Can you work these out from the model? Positions are in its coordinate system, mm. Face numbers are marked on the shaded views. A direction names the side the tool comes from. Round coordinates to 2 decimals unless told otherwise and drop trailing zeros. Write each loop counter-clockwise with the first axis right and the second up, starting at its lowest first coordinate (ties: lowest second). Pieces come first, ordered by that corner, then holes.
Q1. If we section it at C-C (z = 37): Please give me the cut outline in (x, y).
Q2. I'm going to push flat-ended pins straight in: pin 1 Ø19 at (x, y) = (12.5, -7) entering from +Z; pin 2 Ø4 at (x, y) = (-9, 20) entering from -Z; pin 3 Ø2 at (x, y) = (-31, -3.5) entering from +Z; pin 4 Ø8 at (x, y) = (13.5, 2.5) entering from +Z. Where does each tip first touch, or does it pass through?
Q3. Please list where these lines run through material, in increasing order: line 1 along Y through (x, z) = (-7, 8); line 2 along Y through (x, z) = (-3, 14); line 3 along X through (y, z) = (-17, 37.5).
Q4. For the marked faces 1 and 2, which set-ups out of +Z, -Z, +X, -X, +Y, -Y let a thin tool reach every point of the face, with its end or its side?
Q5. If we section it at D-D (x = -20.5): Please give me the cut outline in (y, z).
Q6. If we section it at A-A (x = 0): Please give me the cut outline in (y, z).
Q7. If we section it at B-B (y = 0): Please give me the cut outline in (x, z), plus the area to 3 significant figures.
from build123d import *

# Parameters (mm, degrees)
BOSS_EXTRUDE1_DEPTH = 40
FILLET1_R           = 4
SKETCH2_R           = 30
BOSS_EXTRUDE2_DEPTH = 4
SKETCH3_R           = 13.5
BOSS_EXTRUDE3_DEPTH = 44.5


with BuildPart() as part:
    # Sketch1 → Boss-Extrude1 (new, symmetric)
    with BuildSketch(Plane(origin=(0, 0, 0), x_dir=(0, 0, -1), z_dir=(1, 0, 0))):
        Polygon((0, 32), (0, -32), (11.5, -32), (8, 32), align=None)
    extrude(amount=BOSS_EXTRUDE1_DEPTH, both=True)

    # Fillet1
    fillet1_edges = [part.edges().sort_by_distance(p)[0] for p in [
        (40, -32, -5.75),
        (40, 32, -4),
        (-40, -32, -5.75),
        (-40, 32, -4),
    ]]
    fillet(fillet1_edges, radius=FILLET1_R)

    # Sketch2 → Boss-Extrude2 (add)
    with BuildSketch(Plane.XY):
        with Locations(Location((0, 0, 0), (0, 0, 180))):
            Circle(SKETCH2_R)
    extrude(amount=BOSS_EXTRUDE2_DEPTH)

    # Sketch3 → Boss-Extrude3 (add)
    with BuildSketch(Plane.XY.offset(4)):
        with Locations(Location((0, -17, 0), (0, 0, 249.082562466))):
            Circle(SKETCH3_R)
    extrude(amount=BOSS_EXTRUDE3_DEPTH)


solid = part.part
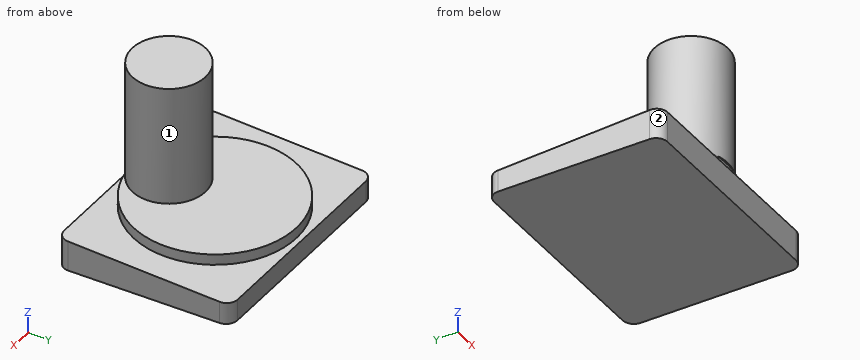
A:
1. outline: circle Ø27 at (0, -17)
2. pin 1: stops at z = 48.5
2. pin 2: stops at z = -8.77
2. pin 3: stops at z = 0
2. pin 4: stops at z = 4
3. line 1: y = -28.54 to -5.46
3. line 2: y = -30.16 to -3.84
3. line 3: x = -13.5 to 13.5
4. face 1: +Z
4. face 2: +Z, -Z, -X, -Y
5. outline: (-32, -11.5) - (32, -8) - (32, 0) - (21.9, 0) - (21.9, 4) - (-21.9, 4) - (-21.9, 0) - (-32, 0) - close
6. outline: (-32, -11.5) - (32, -8) - (32, 0) - (30, 0) - (30, 4) - (-3.5, 4) - (-3.5, 48.5) - (-30.5, 48.5) - (-30.5, 4) - (-30, 4) - (-30, 0) - (-32, 0) - close
7. outline: (-40, -9.75) - (40, -9.75) - (40, 0) - (30, 0) - (30, 4) - (-30, 4) - (-30, 0) - (-40, 0) - close
7. area: 1,020 mm2
